from build123d import *

# Parameters (mm, degrees)
SKETCH3_W          = 2
SKETCH3_H          = 10.621146273
CUT_EXTRUDE1_DEPTH = 10
CIRPATTERN1_COUNT  = 6


with BuildPart() as part:
    # Sketch1 → Revolve1 (revolve)
    with BuildSketch(Plane.XY, mode=Mode.PRIVATE) as revolve1_sk:
        with BuildLine():
            Line((12.7, -3.253426841), (13.447114034, -3.253426841))
            Line((13.447114034, -3.253426841), (13.563291986, 8.746573159))
            Line((13.563291986, 8.746573159), (11.473793749, 18.442570525))
            ThreePointArc((11.473793749, 18.442570525), (10.949794816, 19.29361987), (10.007456249, 19.626573159))
            Line((10.007456249, 19.626573159), (9.5, 19.626573159))
            Line((9.5, 19.626573159), (9.65, 6.746573159))
            Line((9.65, 6.746573159), (12.7, 6.746573159))
            Line((12.7, 6.746573159), (12.7, -3.253426841))
        make_face()
    revolve(revolve1_sk.sketch.rotate(Axis((0, 0, 0), (0, 1, 0)), 90), axis=Axis((0, 0, 0), (0, 1, 0)))

    # Sketch3 → Cut-Extrude1 (cut)
    with BuildSketch(Plane(origin=(0, 19.626573159, 0), x_dir=(1, 0, 0), z_dir=(0, 1, 0))):
        with Locations((0, 10.007456249)):
            Rectangle(SKETCH3_W, SKETCH3_H)
    cut_extrude1 = extrude(amount=-CUT_EXTRUDE1_DEPTH, mode=Mode.SUBTRACT)

    # CirPattern1: Cut-Extrude1 ×6 about axis
    cirpattern1_axis = Axis((0, 0, 0), (0, 1, 0))
    for i in range(1, CIRPATTERN1_COUNT):
        add(cut_extrude1.rotate(cirpattern1_axis, i * 360 / CIRPATTERN1_COUNT), mode=Mode.SUBTRACT)


solid = part.part
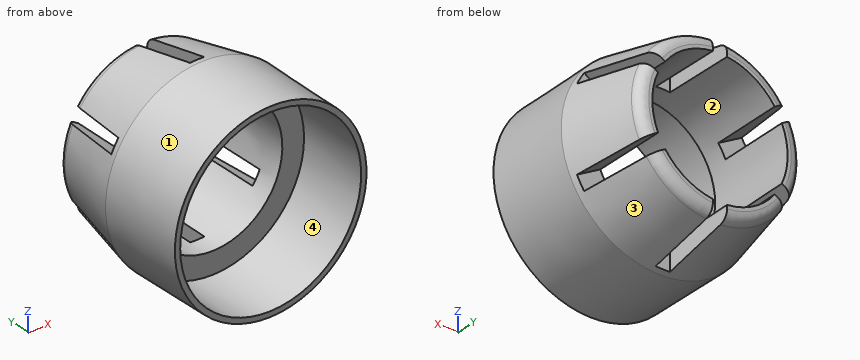
Verification items for the finished model (mm, model axes). Face numbers are marked on the shaded views. A direction names the side the tool comes from. Coordinates: 2 decimals unless noted, no trailing zeros. Order: outer loops, then holes, each group sorted by start corner. A loop starts at its lowest first (then second) coordinate and runs counter-clockwise, first axis right, second up.
Item 1: Release check for a two-part mould opening along X. For the marked faces 1 and 2 record: +X half, -X half, draft (parallel to the pull), parting line (faces both ways), or undercut.
Filled in:
face 1: parting line
face 2: undercut
Item 2: Section check A-A, the plane y = 18. Enter the section's corners in (x, z), then the cut area to 3 significant figures.
Filled in:
outline: (-10.48, -4.9) - (-8.7, -3.87) arc R9.52 cw to (-8.7, 3.87) - (-10.48, 4.9) arc R11.57 ccw to start; (-9.48, -6.63) arc R11.57 ccw to (-1, -11.53) - (-1, -9.47) arc R9.52 cw to (-7.7, -5.6) - close; (-9.48, 6.63) - (-7.7, 5.6) arc R9.52 cw to (-1, 9.47) - (-1, 11.53) arc R11.57 ccw to start; (1, -11.53) arc R11.57 ccw to (9.48, -6.63) - (7.7, -5.6) arc R9.52 cw to (1, -9.47) - close; (1, 9.47) arc R9.52 cw to (7.7, 5.6) - (9.48, 6.63) arc R11.57 ccw to (1, 11.53) - close; (8.7, -3.87) - (10.48, -4.9) arc R11.57 ccw to (10.48, 4.9) - (8.7, 3.87) arc R9.52 cw to start
area: 111 mm2
Item 3: Section check B-B, the plane y = 10.75. Enter the section's corners in (x, z), then the cut area to 3 significant figures.
Filled in:
outline: (-11.84, -5.68) - (-8.77, -3.91) arc R9.6 cw to (-8.77, 3.91) - (-11.84, 5.68) arc R13.13 ccw to start; (-10.84, -7.41) arc R13.13 ccw to (-1, -13.09) - (-1, -9.55) arc R9.6 cw to (-7.77, -5.64) - close; (-10.84, 7.41) - (-7.77, 5.64) arc R9.6 cw to (-1, 9.55) - (-1, 13.09) arc R13.13 ccw to start; (1, -13.09) arc R13.13 ccw to (10.84, -7.41) - (7.77, -5.64) arc R9.6 cw to (1, -9.55) - close; (1, 9.55) arc R9.6 cw to (7.77, 5.64) - (10.84, 7.41) arc R13.13 ccw to (1, 13.09) - close; (8.77, -3.91) - (11.84, -5.68) arc R13.13 ccw to (11.84, 5.68) - (8.77, 3.91) arc R9.6 cw to start
area: 210 mm2
Item 4: Material ranges on L1, parallel to X at y = 3, z = 0; L2, parallel to Z at x = -2.75, y = 18.5; L3, parallel to Z at x = 0.25, y = 0.75, recorded low to high.
Filled in:
L1: x = -13.51 to -12.7, 12.7 to 13.51
L2: z = -11.13 to -9.11, 9.11 to 11.13
L3: z = -13.48 to -12.7, 12.7 to 13.48
Item 5: Depth check by flat-ended pin: pin 1 (3 mm diameter, centred on x = -10, z = 5.5, fed in from +Y); pin 2 (2 mm diameter, centred on x = -0.5, z = -7.5, fed in from +Y); pin 3 (4 mm diameter, centred on x = -10, y = 4, fed in from +Z); pin 4 (1.2 mm diameter, centred on y = 16.5, z = 11.5, fed in from +X). Enter the tip coordinate at first touch or a pass-through.
Filled in:
pin 1: stops at y = 19.62
pin 2: passes through
pin 3: stops at z = 10.9
pin 4: stops at x = 4.79
Item 6: Section check D-D, the plane y = 1.5. Enter the section's corners in (x, z).
Filled in:
outline: circle Ø26.99 at (0, 0); hole circle Ø25.4 at (0, 0)
Item 7: Access from +Z, -Z, +X, -X, +Y, -Y to the whole of each face (thin tool, end or side, straight path). Record for the marked faces 3 and 4.
Filled in:
face 3: +Y
face 4: -Y
